Model file for the job. Use its own axes, mm. A direction names the side the tool comes from. Give positions to 0.01 mm unless a question says otherwise; leave off trailing zeros. Loops run counter-clockwise (first coordinate to the right, second up) from the corner with the lowest first, then second, coordinate; pieces in that order, holes last. Notation, with made-up numbers: M -34.5,41.5 L -18.5,41.5 A25 ccw -18.5,66.5 Z; hole C 13,61.25 d3. An arc over 180 degrees is marked long. Answer in a Markdown table with one row per item.
```python
from build123d import *

# Parameters (mm, degrees)
SKETCH1_R           = 2.75
BOSS_EXTRUDE1_DEPTH = 13.5
SKETCH3_R           = 1.5
BOSS_EXTRUDE2_DEPTH = 1
FILLET1_R           = 0.5
BOSS_EXTRUDE3_START = 1
SKETCH4_R           = 1.5
BOSS_EXTRUDE3_DEPTH = 1
FILLET2_R           = 0.5


with BuildPart() as part:
    # Sketch1 → Boss-Extrude1 (new body)
    with BuildSketch(Plane.XY):
        Circle(SKETCH1_R)
    extrude(amount=BOSS_EXTRUDE1_DEPTH)

    # Sketch3 → Boss-Extrude2 (add)
    with BuildSketch(Plane.XY.offset(13.5)):
        Circle(SKETCH3_R)
    extrude(amount=BOSS_EXTRUDE2_DEPTH)

    # Fillet1
    fillet1_edges = [part.edges().sort_by_distance(p)[0] for p in [
        (-1.5, 0, 14.5),
    ]]
    fillet(fillet1_edges, radius=FILLET1_R)

    # Sketch4 → Boss-Extrude3 (add)
    with BuildSketch(Plane(origin=(0, 0, 0), x_dir=(-1, 0, 0), z_dir=(0, 0, -1)).offset(BOSS_EXTRUDE3_START)):
        with Locations(Location((0, 0, 0), (0, 0, 180))):
            Circle(SKETCH4_R)
    extrude(amount=-BOSS_EXTRUDE3_DEPTH)

    # Fillet2
    fillet2_edges = [part.edges().sort_by_distance(p)[0] for p in [
        (-1.5, 0, -1),
    ]]
    fillet(fillet2_edges, radius=FILLET2_R)


solid = part.part
```
(1) Which spindle directions (+Z, -Z, +X, -X, +Y, -Y) get a long thin tool onto all of the face, cutting with end or side? Do faces 1 (the cylindrical face through (-0.596, -2.685, 6.656)), 2 (the flat face through (1.2, -1.2, 0)), 3 (the cylindrical face through (-1.5, 0.07, 13.75)). Say none if no direction does.
Established:
| item | result |
|---|---|
| face 1 | +Z, -Z |
| face 2 | -Z |
| face 3 | +Z |
(2) Wall check: L1, parallel to Z at x = 1.7, y = -1.5; L2, parallel to X at y = 0.1, z = 0.5. Give the ranges that are in metal, low to high.
Established:
| item | result |
|---|---|
| L1 | z = 0 to 13.5 |
| L2 | x = -2.75 to 2.75 |
(3) Saw through at A-A, the plane y = 0. Give the cut face in (x, z).
Established:
| item | result |
|---|---|
| outline | M -2.75,0 L -1.5,0 L -1.5,-0.5 A0.5 ccw -1,-1 L 1,-1 A0.5 ccw 1.5,-0.5 L 1.5,0 L 2.75,0 L 2.75,13.5 L 1.5,13.5 L 1.5,14 A0.5 ccw 1,14.5 L -1,14.5 A0.5 ccw -1.5,14 L -1.5,13.5 L -2.75,13.5 Z |
(4) Saw through at C-C, the plane z = 9.5. Give the cut face in (x, y), and give its area (3 significant figures).
Established:
| item | result |
|---|---|
| outline | C 0,0 d5.5 |
| area | 23.8 mm2 |
(5) Saw through at D-D, the plane x = 2.45. Give the cut face in (y, z).
Established:
| item | result |
|---|---|
| outline | M -1.25,0 L 1.25,0 L 1.25,13.5 L -1.25,13.5 Z |
